Can you work these out from the model? Positions are in its coordinate system, mm. A direction names the side the tool comes from. Coordinates: 2 decimals unless noted, no trailing zeros. Loops run counter-clockwise (first coordinate to the right, second up) from the corner with the lowest first, then second, coordinate; pieces in that order, holes last.
```python
from build123d import *

# Parameters (mm, degrees)
F1_DEPTH = 762
F3_DEPTH = 762
F4_W     = 707.107375
F4_H     = 601.085796
F5_DEPTH = 1.5875
F6_R     = 304.8
F7_R     = 76.2
F8_R     = 152.4


with BuildPart() as f1:
    # F0 (on Right) → F1 (new body)
    with BuildSketch(Plane.YZ):
        with BuildLine():
            ThreePointArc((0, -347.440392), (-25.4, -372.840392), (0, -398.240392))
            ThreePointArc((0, -398.240392), (152.4, -367.926147), (281.598482, -281.598482))
            ThreePointArc((281.598482, -281.598482), (144.596734, -330.76089), (0, -347.440392))
        make_face()
    extrude(amount=F1_DEPTH)



with BuildPart() as f3:
    # F2 (on Right) → F3 (new body)
    with BuildSketch(Plane.YZ):
        with BuildLine():
            ThreePointArc((196.133325, -181.509551), (178.172813, -212.61807), (209.281333, -230.578583))
            ThreePointArc((209.281333, -230.578583), (305.886805, -182.938036), (376.907375, -101.954596))
            ThreePointArc((376.907375, -101.954596), (289.564758, -148.649932), (196.133325, -181.509551))
        make_face()
    extrude(amount=F3_DEPTH)


with BuildPart() as f1_1:
    add(f1.part)

    add(f3.part)  # F5 merges F3
    # F4 (on face) → F5 (join, symmetric)
    with BuildSketch(Plane.YZ.offset(762)):
        with Locations((175.753688, -250.097494)):
            Rectangle(F4_W, F4_H)
        with BuildLine():
            ThreePointArc((0, -347.440392), (144.596734, -330.76089), (281.598482, -281.598482))
            ThreePointArc((281.598482, -281.598482), (152.4, -367.926147), (0, -398.240392))
            ThreePointArc((0, -398.240392), (-25.4, -372.840392), (0, -347.440392))
        make_face(mode=Mode.SUBTRACT)
        with BuildLine():
            ThreePointArc((0, -398.240392), (152.4, -367.926147), (281.598482, -281.598482))
            ThreePointArc((281.598482, -281.598482), (144.596734, -330.76089), (0, -347.440392))
            ThreePointArc((0, -347.440392), (-25.4, -372.840392), (0, -398.240392))
        make_face()
    extrude(amount=F5_DEPTH, both=True)

    # F6
    f6_edges = [f1_1.edges().sort_by_distance(p)[0] for p in [
        (762, -177.8, 50.445404),
    ]]
    fillet(f6_edges, radius=F6_R)

    # F7
    f7_edges = [f1_1.edges().sort_by_distance(p)[0] for p in [
        (762, -177.8, -550.640392),
        (762, 529.307375, 50.445404),
    ]]
    fillet(f7_edges, radius=F7_R)

    # F8
    f8_edges = [f1_1.edges().sort_by_distance(p)[0] for p in [
        (762, 529.307375, -550.640392),
    ]]
    fillet(f8_edges, radius=F8_R)


solid = f1_1.part
```
(1) If we mould it in two halves opening along Z, with no side actions, what happens to faces 1 (the cylindrical face through (761.98, -90.88, -41.21)), 2 (the cylindrical face through (374.883, 178.034, -212.077)), 3 (the cylindrical face through (762.02, 483.48, -507.18)), 4 (the cylindrical face through (374.883, 146.585, -330.293))? For each: released by +Z, released by -Z, zero draft, split by the parting line, or undercut.
Check values:
face 1: released by +Z
face 2: undercut
face 3: released by -Z
face 4: undercut
(2) I want a section at A-A on x = 340. Write out the boundary of the cut face in (y, z), then the cut area to 3 significant figures.
Check values:
outline: (0, -398.24) arc R398.24 ccw to (281.6, -281.6) arc R635.1 cw to (0, -347.44) arc R25.4 ccw to start; (196.13, -181.51) arc R25.4 ccw to (209.28, -230.58) arc R276.06 ccw to (376.91, -101.95) arc R648.92 cw to start
area: 19,100 mm2
(3) I want a section at C-C on z = -90. Write out the boundary of the cut face in (x, y), then the cut area to 3 significant figures.
Check values:
outline: (760.41, -129.69) - (763.59, -129.69) - (763.59, 529.31) - (760.41, 529.31) - close
area: 2,090 mm2
(4) I want a section at B-B on y = 294.5. Write out the boundary of the cut face in (x, z).
Check values:
outline: (0, -191.22) - (760.41, -191.22) - (760.41, -550.64) - (763.59, -550.64) - (763.59, 50.45) - (760.41, 50.45) - (760.41, -146.45) - (0, -146.45) - close
(5) Which directions (+Z, -Z, +X, -X, +Y, -Y) give clear straight access to the entire face, cutting with the end or side of a thin tool? Please do faces 5 (the cylindrical face through (374.88, 290.83, -148.09)), 6 (the cylindrical face through (374.88, 150.37, -368.76)), 7 (the cylindrical face through (374.883, -25.394, -372.282)).
Check values:
face 5: +Z, -X, -Y
face 6: -Z, -X, +Y
face 7: -X, -Y
(6) If I drill on probe 1 along X at (y, z) = (21, -437); probe 2 along Y at (x, z) = (210, -104); probe 3 along Z at (x, y) = (286, 324.5), over which ranges is the centre line in solid material (lowest first)?
Check values:
probe 1: x = 760.41 to 763.59
probe 2: y = 373.68 to 375.71
probe 3: z = -167.31 to -132.02
(7) I'm going to push flat-ended pins straight in: pin 1 (2 mm diameter, centred on y = -96, z = -103, fed in from -X); pin 2 (10 mm diameter, centred on x = 85, z = -326, fed in from +Y); pin 3 (10 mm diameter, centred on x = 142, y = 261.5, fed in from +Z). Where does each tip first touch, or does it pass through?
Check values:
pin 1: stops at x = 760.41
pin 2: stops at y = 235.7
pin 3: stops at z = -158.27
(8) I want a section at D-D on y = 222. Write out the boundary of the cut face in (x, z).
Check values:
outline: (0, -330.62) - (760.41, -330.62) - (760.41, -550.64) - (763.59, -550.64) - (763.59, 50.45) - (760.41, 50.45) - (760.41, -174) - (0, -174) - (0, -226.84) - (760.41, -226.84) - (760.41, -307.38) - (0, -307.38) - close
